Design review of the part built by this model. Coordinates are the model's own, in mm. Face numbers are marked on the shaded views. A direction names the side the tool comes from. Coordinates: 2 decimals unless noted, no trailing zeros. Loops run counter-clockwise (first coordinate to the right, second up) from the corner with the lowest first, then second, coordinate; pieces in that order, holes last. Notation, with made-up numbers: (-10.75, 57) -> (39.25, 57) arc R29 ccw to (39.25, 77) -> close; hole circle Ø7 at (-24.5, 28.25). An arc over 180 degrees is marked (long way). One line per item, written item: value. Start each with the question number.
1. For probe 1 along Y at (x, z) = (0, 20); probe 2 along X at (y, z) = (384, 59.5); probe 3 along X at (y, z) = (-160, 29), list the stretches that pass through material, from the lowest coordinate up.
2. Add section D-D on x = -584.5. Write out the cut boundary in (y, z), plus the area to 3 significant figures.
3. Add section A-A on z = -481.5. Write out the cut boundary in (x, y), plus the area to 3 significant figures.
4. Machinability: for the marked faces 5, 6, 7, 8 and 9, which of the approach directions +Z, -Z, +X, -X, +Y, -Y give a long, thin tool a straight path to every point of the face, cutting with its end or side? Answer none if there is none.
5. Insertion check: pin 1 (6 mm diameter, centred on y = -288, z = -363.5, fed in from -X); pin 2 (12 mm diameter, centred on x = 567.5, y = 198.5, fed in from +Z); pin 3 (12 mm diameter, centred on x = 552.5, y = 10, fed in from -Z). Each pin has a flat end and moves straight along its axis. Give the tip position at first contact, or say it passes through.
6. Add section B-B on x = 12.5. Write out the cut boundary in (y, z), plus the area to 3 significant figures.
7. Draft analysis for pull direction X (two halves, no side actions). For the marked faces 1, 2, 3 and 4, state which applies: pulls with the +X half, pulls with the -X half, needs draft (parallel to the pull), parting line crosses it, or undercut.
```python
from build123d import *

# Parameters (mm, degrees)
F1_DEPTH  = 100
F5_DEPTH  = 250
F7_DEPTH  = 130
F8_R      = 160
F9_DEPTH  = 480.001
F11_DEPTH = 900
F13_DEPTH = 896.216686194
F15_R     = 190
F15_R_2   = 100
F16_DEPTH = 160
F17_DEPTH = 1230.001
F19_R     = 190
F19_R_2   = 100
F20_DEPTH = 160


with BuildPart() as f1:
    # F0 (on Top) → F1 (new body)
    with BuildSketch(Plane.XY):
        with BuildLine():
            Line((750, 440), (-750, 440))
            Line((-750, 440), (-750, 340))
            Line((-750, 340), (-690, 340))
            ThreePointArc((-690, 340), (-647.5735931288, 322.4264068712), (-630, 280))
            Line((-630, 280), (-630, 72.3790007724))
            ThreePointArc((-630, 72.3790007724), (-604.8683298051, -1.1056915111), (-540, -43.8104996138))
            ThreePointArc((-540, -43.8104996138), (-475.1316701949, -86.5153077165), (-450, -160))
            Line((-450, -160), (-450, -440))
            Line((-450, -440), (450, -440))
            Line((450, -440), (450, -160))
            ThreePointArc((450, -160), (475.1316701949, -86.5153077165), (540, -43.8104996138))
            ThreePointArc((540, -43.8104996138), (604.8683298051, -1.1056915111), (630, 72.3790007724))
            Line((630, 72.3790007724), (630, 280))
            ThreePointArc((630, 280), (647.5735931288, 322.4264068712), (690, 340))
            Line((690, 340), (750, 340))
            Line((750, 340), (750, 440))
        make_face()
    extrude(amount=-F1_DEPTH)

    # F4 (on face) → F5 (join)
    with BuildSketch(Plane.XY):
        with BuildLine():
            Line((410, 340), (750, 340))
            Line((750, 340), (750, 440))
            Line((750, 440), (250, 440))
            Line((250, 440), (250, 220))
            ThreePointArc((250, 220), (241.2132034356, 198.7867965644), (220, 190))
            Line((220, 190), (0, 190))
            Line((0, 190), (-220, 190))
            ThreePointArc((-220, 190), (-241.2132034356, 198.7867965644), (-250, 220))
            Line((-250, 220), (-250, 440))
            Line((-250, 440), (-750, 440))
            Line((-750, 440), (-750, 340))
            Line((-750, 340), (-410, 340))
            ThreePointArc((-410, 340), (-367.5735931288, 322.4264068712), (-350, 280))
            Line((-350, 280), (-350, 210))
            ThreePointArc((-350, 210), (-321.6515138991, 132.5403330759), (-250, 91.678404338))
            Line((-250, 91.678404338), (-250, -160))
            ThreePointArc((-250, -160), (0, -410), (250, -160))
            Line((250, -160), (250, 91.678404338))
            ThreePointArc((250, 91.678404338), (321.6515138991, 132.5403330759), (350, 210))
            Line((350, 210), (350, 280))
            ThreePointArc((350, 280), (367.5735931288, 322.4264068712), (410, 340))
        make_face()
    extrude(amount=F5_DEPTH)

    # F6 (on face) → F7 (join)
    with BuildSketch(Plane.XY.offset(250)):
        with BuildLine():
            ThreePointArc((-250, -160), (0, -410), (250, -160))
            ThreePointArc((250, -160), (0, 90), (-250, -160))
        make_face()
    extrude(amount=F7_DEPTH)

    # F8 (on face) → F9 (cut, through all)
    with BuildSketch(Plane.XY.offset(380)):
        with Locations((0, -160)):
            Circle(F8_R)
    extrude(amount=-F9_DEPTH, mode=Mode.SUBTRACT)

    # F10 (on offset) → F11 (join)
    with BuildSketch(Plane.YZ.offset(450)):
        with BuildLine():
            Line((440, -100), (-440, -100))
            Line((-440, -100), (-416.9663321763, -759.5979458326))
            Line((-416.9663321763, -759.5979458326), (-36.9663321763, -760))
            Line((-36.9663321763, -760), (215.1048871839, -240.8112266237))
            ThreePointArc((215.1048871839, -240.8112266237), (307.3297195, -138.1071103788), (440, -100))
        make_face()
    extrude(amount=-F11_DEPTH)

    # F12 (on face) → F13 (cut, through all)
    with BuildSketch(Plane(origin=(0, -442.9519147444, -15.4682217107), x_dir=(1, 0, 0), z_dir=(0, -0.999390827, -0.0348994967))):
        with BuildLine():
            Line((-350, -144.5833041528), (-350, -864.5833041528))
            Line((-350, -864.5833041528), (350, -864.5833041528))
            Line((350, -864.5833041528), (350, -144.5833041528))
            ThreePointArc((350, -144.5833041528), (332.4264068712, -102.1568972816), (290, -84.5833041528))
            Line((290, -84.5833041528), (-290, -84.5833041528))
            ThreePointArc((-290, -84.5833041528), (-332.4264068712, -102.1568972816), (-350, -144.5833041528))
        make_face()
    extrude(amount=-F13_DEPTH, mode=Mode.SUBTRACT)

    # F15 (on offset) → F16 (join)
    with BuildSketch(Plane.YZ.offset(480)):
        with Locations((-226.9663321763, -759.7989729163)):
            Circle(F15_R)
        with Locations((-226.9663321763, -759.7989729163)):
            Circle(F15_R_2, mode=Mode.SUBTRACT)
    extrude(amount=-F16_DEPTH)

    # F15 (on offset) → F17 (cut, through all)
    with BuildSketch(Plane.YZ.offset(480)):
        with Locations((-226.9663321763, -759.7989729163)):
            Circle(F15_R_2)
    extrude(amount=-F17_DEPTH, mode=Mode.SUBTRACT)

    # F19 (on offset) → F20 (join)
    with BuildSketch(Plane(origin=(-480, 0, 0), x_dir=(0, -1, 0), z_dir=(-1, 0, 0))):
        with Locations((226.9663321763, -759.7989729163)):
            Circle(F19_R)
        with Locations((226.9663321763, -759.7989729163)):
            Circle(F19_R_2, mode=Mode.SUBTRACT)
    extrude(amount=-F20_DEPTH)


solid = f1.part
```
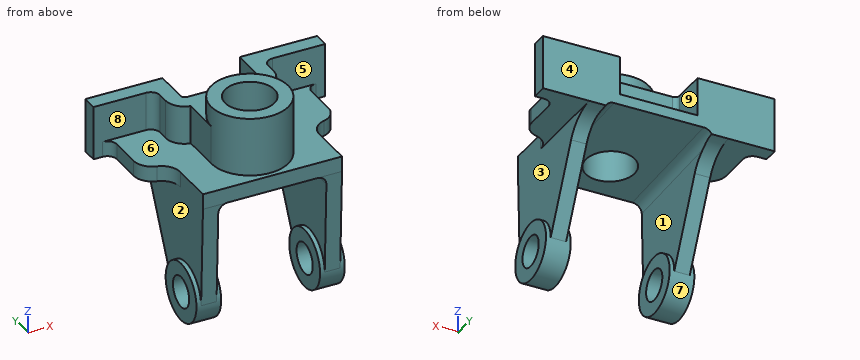
Worked answers:
1. probe 1: y = -410 to -320, 0 to 190
1. probe 2: x = -750 to -250, 250 to 750
1. probe 3: x = -250 to -160, 160 to 250
2. outline: (-21.69, -100) -> (440, -100) -> (440, 250) -> (340, 250) -> (340, 0) -> (-21.69, 0) -> close
2. area: 71,200 mm²
3. outline: (-450, -426.68) -> (-350, -426.68) -> (-350, 98.25) -> (-450, 98.25) -> close; (350, -426.68) -> (450, -426.68) -> (450, 98.25) -> (350, 98.25) -> close
3. area: 105,000 mm²
4. face 5: +Z, +X, -Y
4. face 6: +Z, -Y
4. face 7: none
4. face 8: +Z, -X, -Y
4. face 9: +Z, +Y
5. pin 1: stops at x = -450
5. pin 2: stops at z = 0
5. pin 3: stops at z = -100
6. outline: (-440, -100) -> (-319.51, -95.79) -> (-319.51, 380) -> (-409.69, 380) -> (-409.69, 0) -> (-440, 0) -> close; (-0.49, -84.65) -> (440, -69.27) -> (440, 0) -> (190, 0) -> (190, 250) -> (89.69, 250) -> (89.69, 380) -> (-0.49, 380) -> close
6. area: 139,000 mm²
7. face 1: undercut
7. face 2: pulls with the -X half
7. face 3: pulls with the +X half
7. face 4: needs draft
